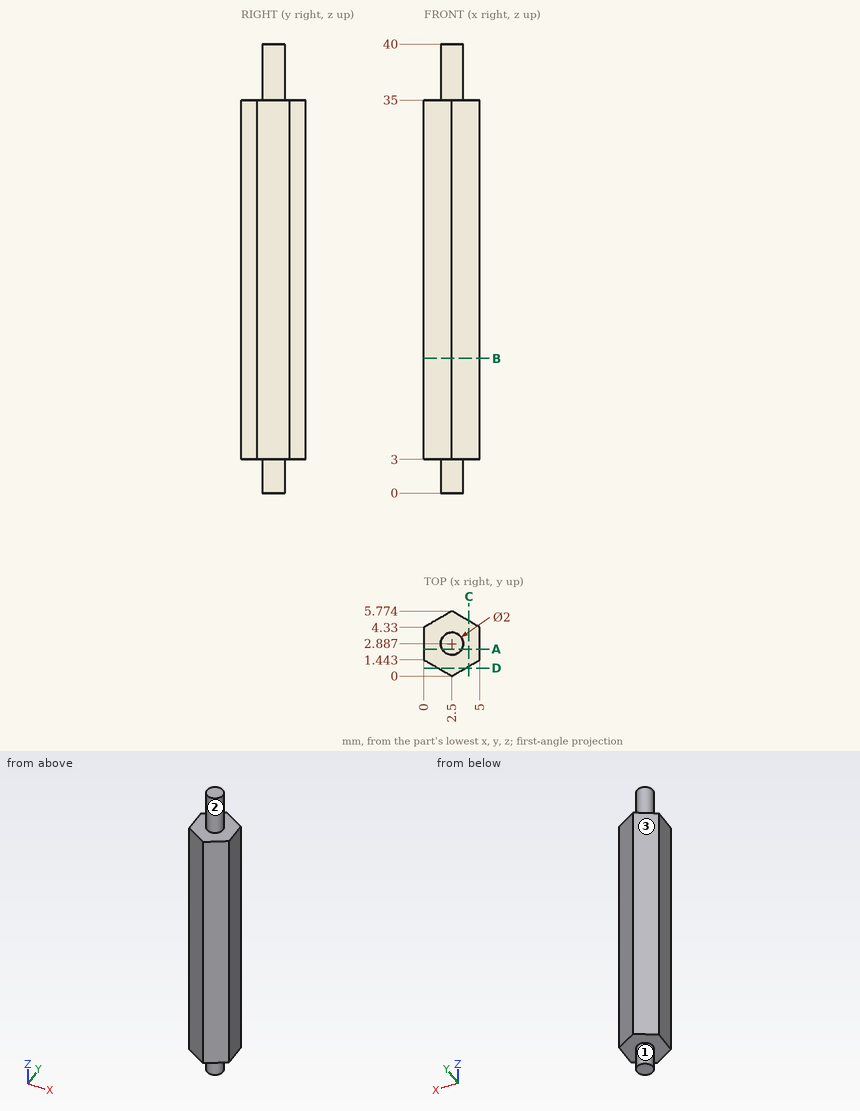
Job drawing, mm, ordinate dimensions from the low corner. One solid piece. A direction names the side the tool comes from. Round coordinates to 2 decimals unless told otherwise and drop trailing zeros. Loops run counter-clockwise (first coordinate to the right, second up) from the corner with the lowest first, then second, coordinate; pieces in that order, holes last.
Item 1: Cut at D-D, the plane y = 0.7. Give the cut face in (x, z).
Item 2: 3-axis set-ups, long thin cutter, end or side, ignore diameter. For the marked faces 1, 2 and 3: which of +Z, -Z, +X, -X, +Y, -Y reach the whole face in a straight line?
Item 3: Cut at C-C, the plane x = 4. Give the cut face in (y, z).
Item 4: Drill centre lines: line 1 (Z direction, x = 1.15, y = 1.3); line 2 (Y direction, x = 3.25, z = 22) (1 decimal); line 3 (X direction, y = 5.5, z = 34.5) (1 decimal). Where is each one in solid material? Low to high.
Item 5: Cut at B-B, the plane z = 12. Give the cut face in (x, y).
Item 6: Cut at A-A, the plane y = 2.4. Give the cut face in (x, z).
A:
1. outline: (1.29, 3) - (3.71, 3) - (3.71, 35) - (1.29, 35) - close
2. face 1: -Z
2. face 2: +Z
2. face 3: +Z, -Z, -X, +Y
3. outline: (0.87, 3) - (4.91, 3) - (4.91, 35) - (0.87, 35) - close
4. line 1: z = 3 to 35
4. line 2: y = 0.4 to 5.3
4. line 3: x = 2 to 3
5. outline: (0, 1.44) - (2.5, 0) - (5, 1.44) - (5, 4.33) - (2.5, 5.77) - (0, 4.33) - close
6. outline: (0, 3) - (1.63, 3) - (1.63, 0) - (3.37, 0) - (3.37, 3) - (5, 3) - (5, 35) - (3.37, 35) - (3.37, 40) - (1.63, 40) - (1.63, 35) - (0, 35) - close
